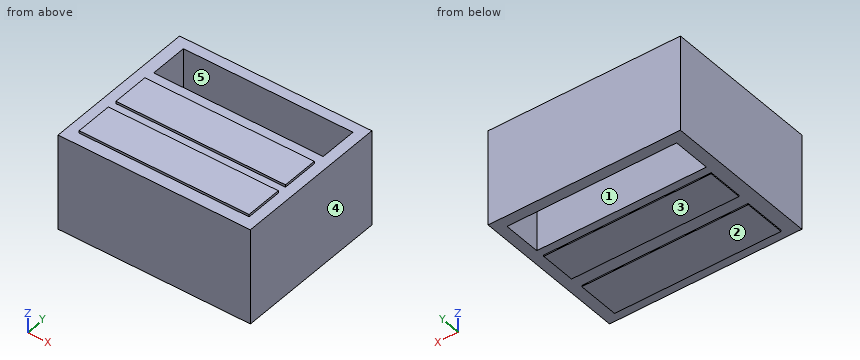
from build123d import *

# Parameters (mm, degrees)
SKETCH_W      = 800
SKETCH_H      = 400
PAD_DEPTH     = 650
SKETCH001_W   = 705.447479
SKETCH001_H   = 159.053192
POCKET_DEPTH  = 400.001
SKETCH002_W   = 696.846951
SKETCH002_H   = 149.011963
SKETCH002_W_2 = 692.598503
SKETCH002_H_2 = 175.711151
PAD001_DEPTH  = 5
SKETCH003_W   = 705.267067
SKETCH003_H   = 154.277191
SKETCH003_W_2 = 707.103642
SKETCH003_H_2 = 156.113739
PAD002_DEPTH  = 10


with BuildPart() as part:
    # Sketch → Pad (new body)
    with BuildSketch(Plane.XZ):
        with Locations((400, 200)):
            Rectangle(SKETCH_W, SKETCH_H)
    extrude(amount=PAD_DEPTH)

    # Sketch001 (on Face1 of Pad) → Pocket (cut, through all)
    with BuildSketch(Plane(origin=(0, 0, 0), x_dir=(1, 0, 0), z_dir=(0, 0, -1))):
        with Locations((402.870193, 123.735901)):
            Rectangle(SKETCH001_W, SKETCH001_H)
    extrude(amount=-POCKET_DEPTH, mode=Mode.SUBTRACT)

    # Sketch002 (on Face1 of Pocket) → Pad001 (join)
    with BuildSketch(Plane(origin=(0, 0, 0), x_dir=(1, 0, 0), z_dir=(0, 0, -1))):
        with Locations((403.497789, 310.137177)):
            Rectangle(SKETCH002_W, SKETCH002_H)
        with Locations((403.533207, 524.328995)):
            Rectangle(SKETCH002_W_2, SKETCH002_H_2)
    extrude(amount=PAD001_DEPTH)

    # Sketch003 (on Face18 of Pad001) → Pad002 (join)
    with BuildSketch(Plane(origin=(0, 0, 400), x_dir=(-1, 0, 0), z_dir=(0, 0, 1))):
        with Locations((-402.754955, 327.754989)):
            Rectangle(SKETCH003_W, SKETCH003_H)
        with Locations((-401.836668, 521.51973)):
            Rectangle(SKETCH003_W_2, SKETCH003_H_2)
    extrude(amount=PAD002_DEPTH)


solid = part.part
The listing builds one solid part. Answer for the finished solid, in the listing's coordinates (mm). Face numbers are marked on the shaded views. A direction names the side the tool comes from. Coordinates: 2 decimals unless noted, no trailing zeros. Loops run counter-clockwise (first coordinate to the right, second up) from the corner with the lowest first, then second, coordinate; pieces in that order, holes last. Notation, with made-up numbers: M 87.25,42.25 L 109.25,42.25 A6 cw 109.25,53.25 Z; hole C -8,48.5 d1. An arc over 180 degrees is marked long. Answer in a Markdown table with one row per item.
1) Given pin 1 (11 mm diameter, centred on y = -325.5, z = 406.5, fed in from -X); pin 2 (2.5 mm diameter, centred on x = 439, z = -2.5, fed in from +Y); pin 3 (5 mm diameter, centred on y = -311, z = 406.5, fed in from +X), each flat-ended and moving along its own axis, determine where each tip first touches the part or whether it passes through.
Answers below:
| item | result |
|---|---|
| pin 1 | x = 50.12 |
| pin 2 | y = -235.63 |
| pin 3 | x = 755.39 |
2) Which of the six approach directions +Z, -Z, +X, -X, +Y, -Y give full straight-line access (tool end or side, diameter ignored) to the marked faces 1 and 2?
Answers below:
| item | result |
|---|---|
| face 1 | +Z, -Z |
| face 2 | -Z, +X, -X, +Y, -Y |
3) Find the intervals of material crossed by probe 1 along Y at (x, z) = (241.5, 69.5); probe 2 along X at (y, z) = (-72.5, 249.5); probe 3 along Z at (x, y) = (570, -401), in increasing order.
Answers below:
| item | result |
|---|---|
| probe 1 | -650 to -203.26, -44.21 to 0 |
| probe 2 | 0 to 50.15, 755.59 to 800 |
| probe 3 | 0 to 410 |
4) Find section B-B (y = -125.5). Determine the outline of the cut face in (x, z), then the cut area to 3 significant figures.
Answers below:
| item | result |
|---|---|
| outline | M 0,0 L 50.15,0 L 50.15,400 L 0,400 Z; M 755.59,0 L 800,0 L 800,400 L 755.59,400 Z |
| area | 37,800 mm^2 |
5) Find section A-A (z = 42.5). Determine the outline of the cut face in (x, y).
Answers below:
| item | result |
|---|---|
| outline | M 0,-650 L 800,-650 L 800,0 L 0,0 Z; hole M 50.15,-203.26 L 755.59,-203.26 L 755.59,-44.21 L 50.15,-44.21 Z |
6) Find section C-C (x = 664). Determine the outline of the cut face in (y, z), then the cut area to 3 significant figures.
Answers below:
| item | result |
|---|---|
| outline | M -650,0 L -612.18,0 L -612.18,-5 L -436.47,-5 L -436.47,0 L -384.64,0 L -384.64,-5 L -235.63,-5 L -235.63,0 L -203.26,0 L -203.26,400 L -250.62,400 L -250.62,410 L -404.89,410 L -404.89,400 L -443.46,400 L -443.46,410 L -599.58,410 L -599.58,400 L -650,400 Z; M -44.21,0 L 0,0 L 0,400 L -44.21,400 Z |
| area | 201,000 mm^2 |
7) Determine the mould class of the marked faces 3, 4 and 5 for opening direction X: released by +X, released by -X, zero draft, split by the parting line, or undercut.
Answers below:
| item | result |
|---|---|
| face 3 | zero draft |
| face 4 | released by +X |
| face 5 | undercut |
